Design review of the part built by this model. Coordinates are the model's own, in mm. Face numbers are marked on the shaded views. Give positions to 0.01 mm unless a question says otherwise; leave off trailing zeros. Loops run counter-clockwise (first coordinate to the right, second up) from the corner with the lowest first, then second, coordinate; pieces in that order, holes last. Notation, with made-up numbers: (20, 72) -> (40, 72) arc R34 ccw to (40, 103) -> close; hole circle Ø7 at (50.5, -3). An arc over 180 degrees is marked (long way). Answer in a Markdown table with one row per item. Add a question column.
(1) Consider section D-D on x = -6.75. Write out the cut boundary in (y, z), then the cut area to 3 significant figures.
(2) Consider section B-B on x = -13.5. Write out the cut boundary in (y, z), then the cut area to 3 significant figures.
(3) For pin 1 (1.8 mm diameter, centred on x = -6.75, y = -11.69, fed in from -Z); pin 2 (1 mm diameter, centred on x = 8.5, y = 12, fed in from +Z); pin 3 (1.5 mm diameter, centred on x = -8, z = -2.5, fed in from -Y); pin 4 (1.5 mm diameter, centred on y = -12, z = -4, fed in from +X), all flat-tipped, find the tip position at first contact; note any pin that passes through.
(4) For line 1 (Y direction, x = -6.75, z = -2.1); line 2 (X direction, y = -14.5, z = -3.4); line 3 (Y direction, x = 3, z = -3.95), list the stretches that pass through material, from the lowest coordinate up.
(5) Consider section C-C on z = -4.6. Write out the cut boundary in (x, y), then the cut area to 3 significant figures.
(6) Consider section A-A on y = 0. Write out the cut boundary in (x, z).
(7) Draft analysis for pull direction X (two halves, no side actions). For the marked faces 1, 2 and 3, state which applies: +X half, -X half, draft (parallel to the pull), parting line (faces both ways), or undercut.
from build123d import *

# Parameters (mm, degrees)
ROTATING_OUTPUT_INTERFACE_START = -5
PROFILE_1_R                     = 17.5
PROFILE_1_R_2                   = 1.52
ROTATING_OUTPUT_INTERFACE_DEPTH = 5


with BuildPart() as part:
    # Profile_1 → Rotating_output_interface (new body)
    with BuildSketch(Plane.XY.offset(ROTATING_OUTPUT_INTERFACE_START)):
        Circle(PROFILE_1_R)
        with Locations((13.5, 0)):
            Circle(PROFILE_1_R_2, mode=Mode.SUBTRACT)
        with Locations((6.75, 11.691342951)):
            Circle(PROFILE_1_R_2, mode=Mode.SUBTRACT)
        with Locations((-6.75, 11.691342951)):
            Circle(PROFILE_1_R_2, mode=Mode.SUBTRACT)
        with Locations((-13.5, 0)):
            Circle(PROFILE_1_R_2, mode=Mode.SUBTRACT)
        with Locations((-6.75, -11.691342951)):
            Circle(PROFILE_1_R_2, mode=Mode.SUBTRACT)
        with Locations((6.75, -11.691342951)):
            Circle(PROFILE_1_R_2, mode=Mode.SUBTRACT)
    extrude(amount=ROTATING_OUTPUT_INTERFACE_DEPTH)


solid = part.part
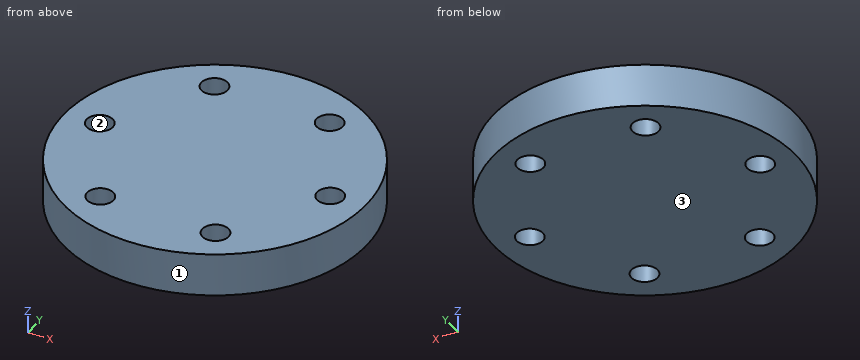
Values follow:
| question | item | result |
|---|---|---|
| 1 | outline | (-16.15, -5) -> (-13.21, -5) -> (-13.21, 0) -> (-16.15, 0) -> close; (-10.17, -5) -> (10.17, -5) -> (10.17, 0) -> (-10.17, 0) -> close; (13.21, -5) -> (16.15, -5) -> (16.15, 0) -> (13.21, 0) -> close |
| 1 | area | 131 mm2 |
| 2 | outline | (-11.14, -5) -> (-1.52, -5) -> (-1.52, 0) -> (-11.14, 0) -> close; (1.52, -5) -> (11.14, -5) -> (11.14, 0) -> (1.52, 0) -> close |
| 2 | area | 96.2 mm2 |
| 3 | pin 1 | through |
| 3 | pin 2 | z = 0 |
| 3 | pin 3 | y = -15.93 |
| 3 | pin 4 | x = 13.4 |
| 4 | line 1 | -16.15 to -13.21, -10.17 to 10.17, 13.21 to 16.15 |
| 4 | line 2 | -9.8 to 9.8 |
| 4 | line 3 | -17.24 to 17.24 |
| 5 | outline | circle Ø35 at (0, 0); hole circle Ø3.04 at (-13.5, 0); hole circle Ø3.04 at (-6.75, -11.69); hole circle Ø3.04 at (-6.75, 11.69); hole circle Ø3.04 at (6.75, -11.69); hole circle Ø3.04 at (6.75, 11.69); hole circle Ø3.04 at (13.5, 0) |
| 5 | area | 919 mm2 |
| 6 | outline | (-17.5, -5) -> (-15.02, -5) -> (-15.02, 0) -> (-17.5, 0) -> close; (-11.98, -5) -> (11.98, -5) -> (11.98, 0) -> (-11.98, 0) -> close; (15.02, -5) -> (17.5, -5) -> (17.5, 0) -> (15.02, 0) -> close |
| 7 | face 1 | parting line |
| 7 | face 2 | undercut |
| 7 | face 3 | draft |
